CAD build for the part. Positions are in the model's coordinates, mm. A direction names the side the tool comes from. Coordinates: 2 decimals unless noted, no trailing zeros. Loops run counter-clockwise (first coordinate to the right, second up) from the corner with the lowest first, then second, coordinate; pieces in that order, holes last. Notation, with made-up numbers: (-2.75, 83.5) -> (29.25, 83.5) arc R26 cw to (29.25, 98.5) -> close; hole circle Ø5 at (51.25, 39). An arc over 180 degrees is marked (long way). Answer as CSV lines item,"result". Start each with the question number.
from build123d import *

# Parameters (mm, degrees)
SKETCH2_W           = 66.5
SKETCH2_H           = 40
BOSS_EXTRUDE1_DEPTH = 5
SKETCH5_W           = 40
SKETCH5_H           = 39
BOSS_EXTRUDE3_DEPTH = 3
SKETCH11_W          = 14.05
SKETCH11_H          = 2.5
SKETCH11_W_2        = 18
SKETCH11_H_2        = 1.5
BOSS_EXTRUDE4_DEPTH = 5.6
FILLET4_R           = 1
FILLET6_R           = 10
SKETCH12_W          = 30
SKETCH12_H          = 40
CUT_EXTRUDE1_DEPTH  = 10
SKETCH13_R          = 10
BOSS_EXTRUDE5_DEPTH = 50
SKETCH14_W          = 40
SKETCH14_H          = 39
BOSS_EXTRUDE6_DEPTH = 3
SKETCH15_W          = 40
SKETCH15_H          = 5
BOSS_EXTRUDE7_DEPTH = 66.5
CUT_EXTRUDE2_DEPTH  = 5


with BuildPart() as part:
    # Sketch2 → Boss-Extrude1 (new body)
    with BuildSketch(Plane(origin=(0, 0, 0), x_dir=(1, 0, 0), z_dir=(0, 1, 0))):
        Rectangle(SKETCH2_W, SKETCH2_H)
        with BuildLine():
            Line((-27.65, 11.5), (-27.65, -11.5))
            ThreePointArc((-27.65, -11.5), (-26.771320344, -13.621320344), (-24.65, -14.5))
            Line((-24.65, -14.5), (28.85, -14.5))
            ThreePointArc((28.85, -14.5), (30.971320344, -13.621320344), (31.85, -11.5))
            Line((31.85, -11.5), (31.85, 11.5))
            ThreePointArc((31.85, 11.5), (30.971320344, 13.621320344), (28.85, 14.5))
            Line((28.85, 14.5), (-24.65, 14.5))
            ThreePointArc((-24.65, 14.5), (-26.771320344, 13.621320344), (-27.65, 11.5))
        make_face(mode=Mode.SUBTRACT)
    extrude(amount=BOSS_EXTRUDE1_DEPTH)

    # Sketch5 → Boss-Extrude3 (add)
    with BuildSketch(Plane.ZY.offset(33.25)):
        with Locations((0, 19.5)):
            Rectangle(SKETCH5_W, SKETCH5_H)
    extrude(amount=BOSS_EXTRUDE3_DEPTH)

    # Sketch11 → Boss-Extrude4 (add)
    with BuildSketch(Plane(origin=(-33.25, 0, 0), x_dir=(0, 0, -1), z_dir=(1, 0, 0))):
        with Locations((0, 35.75)):
            Rectangle(SKETCH11_W, SKETCH11_H)
        with Locations((0, 7.75)):
            Rectangle(SKETCH11_W_2, SKETCH11_H_2)
    extrude(amount=BOSS_EXTRUDE4_DEPTH)

    # Fillet4
    fillet4_edges = [part.edges().sort_by_distance(p)[0] for p in [
        (-27.65, 7.75, -9),
        (-27.65, 7.75, 9),
    ]]
    fillet(fillet4_edges, radius=FILLET4_R)

    # Fillet6
    fillet6_edges = [part.edges().sort_by_distance(p)[0] for p in [
        (33.25, 2.5, 20),
        (33.25, 2.5, -20),
    ]]
    fillet(fillet6_edges, radius=FILLET6_R)

    # Sketch12 → Cut-Extrude1 (cut)
    with BuildSketch(Plane.XZ):
        with Locations((18.25, 0)):
            Rectangle(SKETCH12_W, SKETCH12_H)
    extrude(amount=-CUT_EXTRUDE1_DEPTH, mode=Mode.SUBTRACT)

    # Sketch13 → Boss-Extrude5 (add)
    with BuildSketch(Plane.ZY.offset(36.25)):
        with Locations((0, 19.5)):
            Circle(SKETCH13_R)
    extrude(amount=BOSS_EXTRUDE5_DEPTH)

    # Sketch14 → Boss-Extrude6 (add)
    with BuildSketch(Plane.ZY.offset(86.25)):
        with Locations((0, 19.5)):
            Rectangle(SKETCH14_W, SKETCH14_H)
    extrude(amount=BOSS_EXTRUDE6_DEPTH)

    # Sketch15 → Boss-Extrude7 (add)
    with BuildSketch(Plane.ZY.offset(89.25)):
        with Locations((0, 36.5)):
            Rectangle(SKETCH15_W, SKETCH15_H)
    extrude(amount=BOSS_EXTRUDE7_DEPTH)

    # Sketch16 → Cut-Extrude2 (cut)
    with BuildSketch(Plane.XZ.offset(-34)):
        with BuildLine():
            Line((-152.25, 11.5), (-152.25, -11.5))
            ThreePointArc((-152.25, -11.5), (-151.371320344, -13.621320344), (-149.25, -14.5))
            Line((-149.25, -14.5), (-95.75, -14.5))
            ThreePointArc((-95.75, -14.5), (-93.628679656, -13.621320344), (-92.75, -11.5))
            Line((-92.75, -11.5), (-92.75, 11.5))
            ThreePointArc((-92.75, 11.5), (-93.628679656, 13.621320344), (-95.75, 14.5))
            Line((-95.75, 14.5), (-149.25, 14.5))
            ThreePointArc((-149.25, 14.5), (-151.371320344, 13.621320344), (-152.25, 11.5))
        make_face()
    extrude(amount=-CUT_EXTRUDE2_DEPTH, mode=Mode.SUBTRACT)


solid = part.part
Item 1: Flat gauge pins, fed straight in: pin 1 Ø2.5 at (y, z) = (37, 2.5) entering from +X; pin 2 Ø0.8 at (x, y) = (-31, 35.5) entering from -Z (3 decimals); pin 3 Ø4.5 at (x, z) = (-30.5, -4.5) entering from +Y; pin 4 Ø12 at (x, z) = (-111.5, -8) entering from -Y. Where does each tip first touch, or does it go through?
Item 2: Saw through at A-A (x = -99). Write the cut outline in (y, z).
Item 3: Saw through at B-B (y = 32.5). Write the cut outline in (x, z), plus the area to 3 significant figures.
Item 4: Saw through at C-C (z = 0). Write the cut outline in (x, y), plus the area to 3 significant figures.
Item 5: Which spindle directions (+Z, -Z, +X, -X, +Y, -Y) get a long thin tool onto all of the face, cutting with end or side? Do faces 5 (the face through (-27.65, 2, 0)), 6 (the face through (-36.25, 24.1, -9.2)), 7 (the face through (-118, 39, -15)), 8 (the face through (-30, 7, 0)), 9 (the face through (-93.65, 36.47, -13.64)). Say none if no direction does.
Item 6: Wall check: probe 1 along X at (y, z) = (2.5, 15); probe 2 along X at (y, z) = (28, 12.5); probe 3 along X at (y, z) = (35.5, -14). Give the ranges that are in metal, low to high.
Item 7: Saw through at D-D (y = 19.5). Write the cut outline in (x, z), plus the area to 3 significant figures.
Item 8: Two-plate mould, pull along X, no slides. Class faces 1 (the face through (-89.25, 17, 0)), 2 (the face through (-26.75, 2.46, -13.64)), 3 (the face through (-11, 2, -14.5)), 4 (the face through (-152.25, 36, 0)): pulls with the +X half, pulls with the -X half, needs draft (parallel to the pull), parting line crosses it, or undercut.
Geometry check:
1,pin 1,"x = -27.65"
1,pin 2,"z = -7.025"
1,pin 3,"y = 37"
1,pin 4,"through"
2,outline,"(34, -20) -> (39, -20) -> (39, -14.5) -> (34, -14.5) -> close; (34, 14.5) -> (39, 14.5) -> (39, 20) -> (34, 20) -> close"
3,outline,"(-89.25, -20) -> (-86.25, -20) -> (-86.25, 20) -> (-89.25, 20) -> close; (-36.25, -20) -> (-33.25, -20) -> (-33.25, 20) -> (-36.25, 20) -> close"
3,area,"240 mm2"
4,outline,"(-155.75, 34) -> (-152.25, 34) -> (-152.25, 39) -> (-155.75, 39) -> close; (-92.75, 34) -> (-89.25, 34) -> (-89.25, 0) -> (-86.25, 0) -> (-86.25, 9.5) -> (-36.25, 9.5) -> (-36.25, 0) -> (-27.65, 0) -> (-27.65, 5) -> (-33.25, 5) -> (-33.25, 7) -> (-27.65, 7) -> (-27.65, 8.5) -> (-33.25, 8.5) -> (-33.25, 34.5) -> (-27.65, 34.5) -> (-27.65, 37) -> (-33.25, 37) -> (-33.25, 39) -> (-36.25, 39) -> (-36.25, 29.5) -> (-86.25, 29.5) -> (-86.25, 39) -> (-92.75, 39) -> close"
4,area,"1,320 mm2"
5,face 5,"+X, +Y, -Y"
5,face 6,"none"
5,face 7,"+Z, -Z, +X, -X, +Y"
5,face 8,"+Z, -Z, +X"
5,face 9,"+Y, -Y"
6,probe 1,"-89.25 to -86.25, -36.25 to 3.25"
6,probe 2,"-89.25 to -86.25, -36.25 to -33.25"
6,probe 3,"-155.75 to -150.91, -94.09 to -86.25, -36.25 to -33.25"
7,outline,"(-89.25, -20) -> (-86.25, -20) -> (-86.25, -10) -> (-36.25, -10) -> (-36.25, -20) -> (-33.25, -20) -> (-33.25, 20) -> (-36.25, 20) -> (-36.25, 10) -> (-86.25, 10) -> (-86.25, 20) -> (-89.25, 20) -> close"
7,area,"1,240 mm2"
8,face 1,"pulls with the -X half"
8,face 2,"pulls with the +X half"
8,face 3,"needs draft"
8,face 4,"undercut"
